The model under review builds one solid part; all positions refer to its coordinate system, in mm. Round coordinates to 2 decimals unless told otherwise and drop trailing zeros. Write each loop counter-clockwise with the first axis right and the second up, starting at its lowest first coordinate (ties: lowest second). Pieces come first, ordered by that corner, then holes. Notation, with made-up numbers: (-38, 62.25) -> (-12, 62.25) arc R18 cw to (-12, 90.25) -> close; hole circle Ø10 at (71, 41). An arc over 180 degrees is marked (long way). Return JSON: item names as keys, results as strings. Group by question number.
1. Take a section at A-A, the plane z = 87.5. Write out the cut boundary in (x, y).
2. Clearance check with a flat-ended pin moving along its axis: P1, Ø6, axis at x = 6.35, z = 5.08, coming from the +Y side. State where the tip first meets the part, or that it passes through.
3. For line 1 along Z through (x, y) = (6.35, 2.5) (3 decimals); line 2 along Z through (x, y) = (6, 1.5); line 3 along X through (y, z) = (4, 222.25) (3 decimals), list the stretches that pass through material, from the lowest coordinate up. Write a range as from..to.
Autodesk Inventor part; units mm, degrees
ref_plane "YZ Plane" through (0, 0, 0) normal (1, 0, 0) x (0, 1, 0)
ref_plane "XZ Plane" through (0, 0, 0) normal (0, 1, 0) x (-1, 0, 0)
ref_plane "XY Plane" through (0, 0, 0) normal (0, 0, 1) x (1, 0, 0)
sketch "Sketch1" plane through (0, 0, 0) normal (0, 0, 1) x (1, 0, 0)
  line L0 (0, 0) -> (12.7, 0)
  line L1 (12.7, 0) -> (12.7, 6.35)
  line L2 (12.7, 6.35) -> (0, 6.35)
  line L3 (0, 6.35) -> (0, 0)
  dimension "d0" = 12.7
  dimension "d1" = 6.35
extrude "Extrusion1" add sketch "Sketch1" along normal blind 444.5
chamfer "Chamfer2" distance 1.27 angle 45 12 edges at (12.7, 0, 222.25) (0, 0, 222.25) (12.7, 6.35, 222.25) (0, 6.35, 222.25) (6.35, 0, 444.5) (6.35, 6.35, 444.5) (6.35, 0, 0) (6.35, 6.35, 0) (12.7, 3.175, 0) (0, 3.175, 0) (0, 3.175, 444.5) (12.7, 3.175, 444.5)
sketch "Sketch3" plane through (1.27, 6.35, 1.27) normal (0, 1, 0) x (1, 0, 0)
  line L0 (10.16, 0) -> (10.16, -441.96)
  line L1 (0, 0) -> (10.16, 0)
  line L2 (0, -441.96) -> (10.16, -441.96)
  point P0 (-1.27, 1.27)
  point P1 (5.08, -3.81)
  point P2 (5.08, -220.98)
  point P3 (5.08, -438.15)
  point P4 (22.86, 0)
  point P5 (22.86, -441.96)
  dimension "d17" = 5.08
  dimension "d18" = 3.81
  dimension "d19" = 5.08
  dimension "d20" = 3.81
  dimension "d21" = 5.08
  dimension "d22" = 220.98
hole "Hole1" at (6.35, 6.35, 5.08) at (6.35, 6.35, 222.25) at (6.35, 6.35, 439.42) direction (0, -1, 0) diameter 3.81 end through all
properties part number "x-lift arm prototype piece"
Output:
{
 "1": {"outline": "(0, 1.27) -> (1.27, 0) -> (11.43, 0) -> (12.7, 1.27) -> (12.7, 5.08) -> (11.43, 6.35) -> (1.27, 6.35) -> (0, 5.08) -> close"},
 "2": {"P1": "stops at y = 6.35"},
 "3": {"line 1": "z = 0..3.175, 6.985..220.345, 224.155..437.515, 441.325..444.5", "line 2": "z = 0..3.21, 6.95..220.38, 224.12..437.55, 441.29..444.5", "line 3": "x = 0..4.445, 8.255..12.7"}
}
